```python
from build123d import *

# Parameters (mm, degrees)
RAIL_EXTRUDE_DEPTH = 120
SKETCH2_R          = 0.75
FIRST_HOLE_DEPTH   = 123.068100465
SKETCH3_R          = 0.75
LAST_HOLE_DEPTH    = 123.068100465
ANGLE_DEPTH        = 121.962670283


with BuildPart() as part:
    # Sketch1 → Rail-Extrude (new body)
    with BuildSketch(Plane.XY):
        Polygon((3.991071429, 6.778571429), (6.991071429, 6.778571429), (6.991071429, 0.078571429), (15.291071429, 0.078571429), (15.291071429, 6.778571429), (17.291071429, 6.778571429), (17.291071429, -7.421428571), (3.991071429, -7.421428571), align=None)
    extrude(amount=RAIL_EXTRUDE_DEPTH)

    # Sketch2 → First Hole (cut, through all)
    with BuildSketch(Plane(origin=(0, 6.778571429, 0), x_dir=(1, 0, 0), z_dir=(0, 1, 0))):
        with Locations(Location((5.841071429, -8, 0), (0, 0, 270))):
            Circle(SKETCH2_R)
    extrude(amount=-FIRST_HOLE_DEPTH, mode=Mode.SUBTRACT)

    # Sketch3 → Last Hole (cut, through all)
    with BuildSketch(Plane(origin=(0, 6.778571429, 0), x_dir=(1, 0, 0), z_dir=(0, 1, 0))):
        with Locations(Location((5.841071429, -116, 0), (0, 0, 270))):
            Circle(SKETCH3_R)
    extrude(amount=-LAST_HOLE_DEPTH, mode=Mode.SUBTRACT)

    # Sketch5 → Angle (cut, through all)
    with BuildSketch(Plane.ZY.offset(-3.991071429)):
        Polygon((12.7, -7.421428571), (0, 5.278571429), (0, -7.421428571), align=None)
    extrude(amount=-ANGLE_DEPTH, mode=Mode.SUBTRACT)


solid = part.part
```
Model file for the job. Use its own axes, mm. A direction names the side the tool comes from. Coordinates: 2 decimals unless noted, no trailing zeros. Write each loop counter-clockwise with the first axis right and the second up, starting at its lowest first coordinate (ties: lowest second). Pieces come first, ordered by that corner, then holes. Notation, with made-up numbers: (-7.75, 60) - (41.25, 60) arc R5 ccw to (41.25, 65) - close; hole circle Ø5 at (37, 84.5). An arc over 180 degrees is marked (long way). One line per item, written item: value. Start each with the question number.
1. Probe line 1 (X direction, y = -3, z = 116); line 2 (X direction, y = 4, z = 8); line 3 (X direction, y = 2, z = 50.5). List the from-to ranges inside material, lowest first. Write a range as from..to.
2. Slice it at C-C (y = -1.75). Write the cut outline in (x, z), plus the area to 3 significant figures.
3. Slice it at B-B (z = 72). Write the cut outline in (x, y).
4. Flat gauge pin, fed straight in: pin 1 (3 mm diameter, centred on x = 14, y = 3.5, fed in from -Z). Where does the tip first touch, or does it go through?
5. Tool access for faces 4 (the flat face through (3.991, 0, 59)), 5 (the flat face through (11, 0.079, 62)): list every direction of +Z, -Z, +X, -X, +Y, -Y with a clear straight run to the whole face (end or side of a thin tool).
6. Slice it at A-A (y = 3). Write the cut outline in (x, z).
7. Slice it at D-D (x = 10.25). Write the cut outline in (y, z).
8. Mould opens along Z. For faces 1 (the flat face through (10.55, -2.57, 7.85)), 2 (the flat face through (6.991, 3, 59)), 3 (the flat face through (11, -2, 120)) say: released by +Z, released by -Z, zero draft, split by the parting line, or undercut.
Answers below:
1. line 1: x = 3.99..5.09, 6.59..17.29
1. line 2: x = 3.99..5.09, 6.59..6.99, 15.29..17.29
1. line 3: x = 3.99..6.99, 15.29..17.29
2. outline: (3.99, 7.03) - (17.29, 7.03) - (17.29, 120) - (3.99, 120) - close; hole circle Ø1.5 at (5.84, 8); hole circle Ø1.5 at (5.84, 116)
2. area: 1,500 mm^2
3. outline: (3.99, -7.42) - (17.29, -7.42) - (17.29, 6.78) - (15.29, 6.78) - (15.29, 0.08) - (6.99, 0.08) - (6.99, 6.78) - (3.99, 6.78) - close
4. pin 1: stops at z = 1.01
5. face 4: +Z, -Z, -X, +Y, -Y
5. face 5: +Z, -Z, +Y
6. outline: (3.99, 2.28) - (6.99, 2.28) - (6.99, 120) - (3.99, 120) - close; (15.29, 2.28) - (17.29, 2.28) - (17.29, 120) - (15.29, 120) - close; hole circle Ø1.5 at (5.84, 8); hole circle Ø1.5 at (5.84, 116)
7. outline: (-7.42, 12.7) - (0.08, 5.2) - (0.08, 120) - (-7.42, 120) - close
8. face 1: released by -Z
8. face 2: zero draft
8. face 3: released by +Z
